Design review of the part built by this model. Coordinates are the model's own, in mm. Coordinates: 2 decimals unless noted, no trailing zeros. Write each loop counter-clockwise with the first axis right and the second up, starting at its lowest first coordinate (ties: lowest second). Pieces come first, ordered by that corner, then holes.
Q1. Take a section at C-C (x = 2.5). Give the boundary of the cut face in (y, z).
Q2. Take a section at A-A (z = -10). Give the boundary of the cut face in (x, y), and give its area (3 significant figures).
Q3. Take a section at B-B (y = -1.5). Give the boundary of the cut face in (x, z).
Q4. Insertion check: pin 1 (3 mm diameter, centred on y = -2.5, z = 19.5, fed in from -X); pin 2 (1.5 mm diameter, centred on y = 0.5, z = 8, fed in from +X); pin 3 (3 mm diameter, centred on y = -2, z = -2.5, fed in from +X). Each pin has a flat end and moves straight along its axis. Give the tip position at first contact, or say it passes through.
Q5. For probe 1 along Z at (x, y) = (-50, 1.65); probe 2 along Y at (x, z) = (-19.5, 17.5); probe 3 along X at (y, z) = (-0.5, -2), list the stretches that pass through material, from the lowest coordinate up.
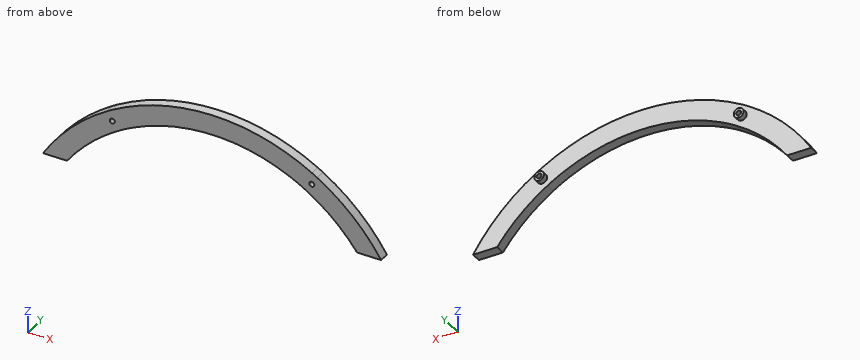
```python
from build123d import *

# Parameters (mm, degrees)
F0_R     = 2.45
F0_R_2   = 1.25
F1_DEPTH = 5
F2_DEPTH = 2.7


with BuildPart() as f1:
    # F0 (on Front) → F1 (new body)
    with BuildSketch(Plane.XZ):
        with BuildLine():
            ThreePointArc((50.0836358252, 13.4458006649), (0, 26.8916013299), (-50.0836358252, 13.4458006649))
            ThreePointArc((-50.0836358252, 13.4458006649), (-48.8562145849, 12.7470900403), (-47.6190477051, 12.0657842722))
            ThreePointArc((-47.6190477051, 12.0657842722), (-43.4045903326, 9.9109244244), (-39.0928846634, 7.9579097983))
            ThreePointArc((-39.0928846634, 7.9579097983), (0, 16.8916013299), (39.0928846634, 7.9579097983))
            ThreePointArc((39.0928846634, 7.9579097983), (43.4045901471, 9.910924335), (47.6190473429, 12.0657840761))
            ThreePointArc((47.6190473429, 12.0657840761), (48.8562144052, 12.7470899397), (50.0836358252, 13.4458006649))
        make_face()
        with BuildLine():
            ThreePointArc((-47.3684207798, 3.4176277054), (-54.2514458754, 5.0374944493), (-52.6315787551, 11.9205194563))
            ThreePointArc((-52.6315787551, 11.9205194563), (-70.5117896256, -2.1993899068), (-84.7319183702, -20))
            Line((-84.7319183702, -20), (-72.6601540784, -20))
            ThreePointArc((-72.6601540784, -20), (-61.1458176612, -7.0690998963), (-47.3684207798, 3.4176277054))
        make_face()
        with BuildLine():
            ThreePointArc((84.7319183702, -20), (70.511789623, -2.1993899042), (52.6315787487, 11.9205194603))
            ThreePointArc((52.6315787487, 11.9205194603), (54.3679453833, 10.1023948559), (55, 7.6690734369))
            ThreePointArc((55, 7.6690734369), (52.4333212381, 3.3011279528), (47.3684208991, 3.4176276316))
            ThreePointArc((47.3684208991, 3.4176276316), (61.1458177127, -7.0690999439), (72.6601540784, -20))
            Line((72.6601540784, -20), (84.7319183702, -20))
        make_face()
        with BuildLine():
            ThreePointArc((-45, 7.6690734369), (-45.7043765601, 10.2279050575), (-47.6190477051, 12.0657842722))
            ThreePointArc((-47.6190477051, 12.0657842722), (-50.1448408517, 12.6669751094), (-52.6315787551, 11.9205194563))
            ThreePointArc((-52.6315787551, 11.9205194563), (-54.2514458754, 5.0374944493), (-47.3684207798, 3.4176277054))
            ThreePointArc((-47.3684207798, 3.4176277054), (-45.6320544817, 5.2357522601), (-45, 7.6690734369))
        make_face()
        with Locations((-50, 7.6690734369)):
            Circle(F0_R, mode=Mode.SUBTRACT)
        with BuildLine():
            ThreePointArc((52.6315787487, 11.9205194603), (50.1448406421, 12.6669751154), (47.6190473429, 12.0657840761))
            ThreePointArc((47.6190473429, 12.0657840761), (45.0020983275, 7.813914286), (47.3684208991, 3.4176276316))
            ThreePointArc((47.3684208991, 3.4176276316), (52.4333212381, 3.3011279528), (55, 7.6690734369))
            ThreePointArc((55, 7.6690734369), (54.3679453833, 10.1023948559), (52.6315787487, 11.9205194603))
        make_face()
        with Locations((50, 7.6690734369)):
            Circle(F0_R, mode=Mode.SUBTRACT)
        with BuildLine():
            ThreePointArc((-39.0928846634, 7.9579097983), (-43.4045903326, 9.9109244244), (-47.6190477051, 12.0657842722))
            ThreePointArc((-47.6190477051, 12.0657842722), (-45.7043765601, 10.2279050575), (-45, 7.6690734369))
            ThreePointArc((-45, 7.6690734369), (-45.6320544817, 5.2357522601), (-47.3684207798, 3.4176277054))
            ThreePointArc((-47.3684207798, 3.4176277054), (-43.2902168521, 5.7963358196), (-39.0928846634, 7.9579097983))
        make_face()
        with BuildLine():
            ThreePointArc((47.3684208991, 3.4176276316), (45.0020983275, 7.813914286), (47.6190473429, 12.0657840761))
            ThreePointArc((47.6190473429, 12.0657840761), (43.4045901471, 9.910924335), (39.0928846634, 7.9579097983))
            ThreePointArc((39.0928846634, 7.9579097983), (43.2902169136, 5.7963357859), (47.3684208991, 3.4176276316))
        make_face()
        with Locations((-50, 7.6690734369)):
            Circle(F0_R)
        with Locations((-50, 7.6690734369)):
            Circle(F0_R_2, mode=Mode.SUBTRACT)
        with Locations((50, 7.6690734369)):
            Circle(F0_R)
        with Locations((50, 7.6690734369)):
            Circle(F0_R_2, mode=Mode.SUBTRACT)
        with BuildLine():
            ThreePointArc((-47.6190477051, 12.0657842722), (-48.8562145849, 12.7470900403), (-50.0836358252, 13.4458006649))
            ThreePointArc((-50.0836358252, 13.4458006649), (-51.363269437, 12.692618531), (-52.6315787551, 11.9205194563))
            ThreePointArc((-52.6315787551, 11.9205194563), (-50.1448408517, 12.6669751094), (-47.6190477051, 12.0657842722))
        make_face()
        with BuildLine():
            ThreePointArc((52.6315787487, 11.9205194603), (51.3632694338, 12.6926185329), (50.0836358252, 13.4458006649))
            ThreePointArc((50.0836358252, 13.4458006649), (48.8562144052, 12.7470899397), (47.6190473429, 12.0657840761))
            ThreePointArc((47.6190473429, 12.0657840761), (50.1448406421, 12.6669751154), (52.6315787487, 11.9205194603))
        make_face()
    extrude(amount=F1_DEPTH)

    # F0 (on Front) → F2 (join)
    with BuildSketch(Plane.XZ):
        with Locations((50, 7.6690734369)):
            Circle(F0_R)
        with Locations((50, 7.6690734369)):
            Circle(F0_R_2, mode=Mode.SUBTRACT)
        with Locations((-50, 7.6690734369)):
            Circle(F0_R)
        with Locations((-50, 7.6690734369)):
            Circle(F0_R_2, mode=Mode.SUBTRACT)
    extrude(amount=-F2_DEPTH)


solid = f1.part
```
Response:
1. outline: (-5, 16.86) - (0, 16.86) - (0, 26.86) - (-5, 26.86) - close
2. outline: (-77.57, -5) - (-64.17, -5) - (-64.17, 0) - (-77.57, 0) - close; (64.17, -5) - (77.57, -5) - (77.57, 0) - (64.17, 0) - close
2. area: 134 mm2
3. outline: (-84.73, -20) - (-72.66, -20) arc R90 cw to (72.66, -20) - (84.73, -20) arc R100 ccw to start; hole circle Ø2.5 at (-50, 7.67); hole circle Ø2.5 at (50, 7.67)
4. pin 1: stops at x = -41.22
4. pin 2: stops at x = 59.26
4. pin 3: stops at x = 72.28
5. probe 1: z = 5.22 to 6.42, 8.92 to 10.12
5. probe 2: y = -5 to 0
5. probe 3: x = -70.31 to -55.17, 55.17 to 70.31
